Work out the finished part from the listing and answer in its coordinate system (mm). Face numbers are marked on the shaded views. Round coordinates to 2 decimals unless told otherwise and drop trailing zeros. Write each loop counter-clockwise with the first axis right and the second up, starting at its lowest first coordinate (ties: lowest second). Pieces come first, ordered by that corner, then holes. Notation, with made-up numbers: (33.5, -3) -> (65.5, -3) arc R19 ccw to (65.5, 21) -> close; hole circle Ø1 at (18, -13). An arc over 180 degrees is marked (long way). One line per item, written item: value.
```python
from build123d import *

# Parameters (mm, degrees)
SKETCH1_R           = 0.5
SKETCH1_R_2         = 0.25
SKETCH1_R_3         = 0.203
SKETCH1_R_4         = 1.25
BOSS_EXTRUDE1_DEPTH = 1.57
SKETCH2_R           = 1.758
SKETCH2_R_2         = 1.25
BOSS_EXTRUDE2_DEPTH = 0.0254
SKETCH3_R           = 0.881
SKETCH3_R_2         = 0.5
BOSS_EXTRUDE3_DEPTH = 0.0254


with BuildPart() as part:
    # Sketch1 → Boss-Extrude1 (new body)
    with BuildSketch(Plane(origin=(0, 0, 0), x_dir=(-1, 0, 0), z_dir=(0, 0, -1))):
        with BuildLine():
            Line((-22.86, 0), (-2.54, 0))
            ThreePointArc((-2.54, 0), (-0.743948776, 0.743948776), (0, 2.54))
            Line((0, 2.54), (0, 20.32))
            ThreePointArc((0, 20.32), (-0.743948776, 22.116051224), (-2.54, 22.86))
            Line((-2.54, 22.86), (-22.86, 22.86))
            ThreePointArc((-22.86, 22.86), (-24.656051224, 22.116051224), (-25.4, 20.32))
            Line((-25.4, 20.32), (-25.4, 2.54))
            ThreePointArc((-25.4, 2.54), (-24.656051224, 0.743948776), (-22.86, 0))
        make_face()
        with Locations(Location((-22.86, 2.54, 0), (0, 0, 180))):
            Circle(SKETCH1_R, mode=Mode.SUBTRACT)
        with Locations(Location((-17.78, 2.54, 0), (0, 0, 180))):
            Circle(SKETCH1_R, mode=Mode.SUBTRACT)
        with Locations(Location((-12.7, 2.54, 0), (0, 0, 180))):
            Circle(SKETCH1_R, mode=Mode.SUBTRACT)
        with Locations(Location((-7.62, 2.54, 0), (0, 0, 180))):
            Circle(SKETCH1_R, mode=Mode.SUBTRACT)
        with Locations(Location((-2.54, 2.54, 0), (0, 0, 180))):
            Circle(SKETCH1_R, mode=Mode.SUBTRACT)
        with Locations(Location((-7.874, 20.32, 0), (0, 0, 180))):
            Circle(SKETCH1_R_2, mode=Mode.SUBTRACT)
        with Locations(Location((-10.922, 15.24, 0), (0, 0, 180))):
            Circle(SKETCH1_R_2, mode=Mode.SUBTRACT)
        with Locations(Location((-11.684, 12.192, 0), (0, 0, 180))):
            Circle(SKETCH1_R_2, mode=Mode.SUBTRACT)
        with Locations(Location((-17.285, 13.462, 0), (0, 0, 180))):
            Circle(SKETCH1_R_3, mode=Mode.SUBTRACT)
        with Locations(Location((-20.828, 18.288, 0), (0, 0, 180))):
            Circle(SKETCH1_R_2, mode=Mode.SUBTRACT)
        with Locations(Location((-5.842, 15.494, 0), (0, 0, 180))):
            Circle(SKETCH1_R_2, mode=Mode.SUBTRACT)
        with Locations(Location((-16.256, 16.002, 0), (0, 0, 180))):
            Circle(SKETCH1_R_2, mode=Mode.SUBTRACT)
        with Locations(Location((-19.558, 13.462, 0), (0, 0, 180))):
            Circle(SKETCH1_R_3, mode=Mode.SUBTRACT)
        with Locations(Location((-11.938, 13.716, 0), (0, 0, 180))):
            Circle(SKETCH1_R_2, mode=Mode.SUBTRACT)
        with Locations(Location((-2.54, 20.32, 0), (0, 0, 180))):
            Circle(SKETCH1_R_4, mode=Mode.SUBTRACT)
        with Locations(Location((-22.86, 20.32, 0), (0, 0, 180))):
            Circle(SKETCH1_R_4, mode=Mode.SUBTRACT)
        with Locations(Location((-5.08, 2.54, 0), (0, 0, 180))):
            Circle(SKETCH1_R, mode=Mode.SUBTRACT)
        with Locations(Location((-10.16, 2.54, 0), (0, 0, 180))):
            Circle(SKETCH1_R, mode=Mode.SUBTRACT)
        with Locations(Location((-15.24, 2.54, 0), (0, 0, 180))):
            Circle(SKETCH1_R, mode=Mode.SUBTRACT)
        with Locations(Location((-20.32, 2.54, 0), (0, 0, 180))):
            Circle(SKETCH1_R, mode=Mode.SUBTRACT)
    extrude(amount=-BOSS_EXTRUDE1_DEPTH)

    # Sketch2 → Boss-Extrude2 (add)
    # profile 1 of 2: a face of its own
    with BuildSketch(Plane.XY.offset(1.57)):
        with Locations(Location((2.54, 20.32, 0), (0, 0, 180))):
            Circle(SKETCH2_R)
        with Locations((2.54, 20.32)):
            Circle(SKETCH2_R_2, mode=Mode.SUBTRACT)
    # profile 2 of 2: a face of its own
    with BuildSketch(Plane.XY.offset(1.57)):
        with Locations(Location((22.86, 20.32, 0), (0, 0, 180))):
            Circle(SKETCH2_R)
        with Locations((22.86, 20.32)):
            Circle(SKETCH2_R_2, mode=Mode.SUBTRACT)
    boss_extrude2 = extrude(amount=BOSS_EXTRUDE2_DEPTH)

    # Mirror1: Boss-Extrude2 across plane
    add(boss_extrude2.mirror(Plane.XY.offset(0.785)))

    # Sketch3 → Boss-Extrude3 (add)
    # profile 1 of 9: a face of its own
    with BuildSketch(Plane.XY.offset(1.57)):
        with Locations(Location((2.54, 2.54, 0), (0, 0, 180))):
            Circle(SKETCH3_R)
        with Locations((2.54, 2.54)):
            Circle(SKETCH3_R_2, mode=Mode.SUBTRACT)
    # profile 2 of 9: a face of its own
    with BuildSketch(Plane.XY.offset(1.57)):
        with Locations(Location((5.08, 2.54, 0), (0, 0, 180))):
            Circle(SKETCH3_R)
        with Locations((5.08, 2.54)):
            Circle(SKETCH3_R_2, mode=Mode.SUBTRACT)
    # profile 3 of 9: a face of its own
    with BuildSketch(Plane.XY.offset(1.57)):
        with Locations(Location((7.62, 2.54, 0), (0, 0, 180))):
            Circle(SKETCH3_R)
        with Locations((7.62, 2.54)):
            Circle(SKETCH3_R_2, mode=Mode.SUBTRACT)
    # profile 4 of 9: a face of its own
    with BuildSketch(Plane.XY.offset(1.57)):
        with Locations(Location((10.16, 2.54, 0), (0, 0, 180))):
            Circle(SKETCH3_R)
        with Locations((10.16, 2.54)):
            Circle(SKETCH3_R_2, mode=Mode.SUBTRACT)
    # profile 5 of 9: a face of its own
    with BuildSketch(Plane.XY.offset(1.57)):
        with Locations(Location((12.7, 2.54, 0), (0, 0, 180))):
            Circle(SKETCH3_R)
        with Locations((12.7, 2.54)):
            Circle(SKETCH3_R_2, mode=Mode.SUBTRACT)
    # profile 6 of 9: a face of its own
    with BuildSketch(Plane.XY.offset(1.57)):
        with Locations(Location((15.24, 2.54, 0), (0, 0, 180))):
            Circle(SKETCH3_R)
        with Locations((15.24, 2.54)):
            Circle(SKETCH3_R_2, mode=Mode.SUBTRACT)
    # profile 7 of 9: a face of its own
    with BuildSketch(Plane.XY.offset(1.57)):
        with Locations(Location((17.78, 2.54, 0), (0, 0, 180))):
            Circle(SKETCH3_R)
        with Locations((17.78, 2.54)):
            Circle(SKETCH3_R_2, mode=Mode.SUBTRACT)
    # profile 8 of 9: a face of its own
    with BuildSketch(Plane.XY.offset(1.57)):
        with Locations(Location((20.32, 2.54, 0), (0, 0, 180))):
            Circle(SKETCH3_R)
        with Locations((20.32, 2.54)):
            Circle(SKETCH3_R_2, mode=Mode.SUBTRACT)
    # profile 9 of 9: a face of its own
    with BuildSketch(Plane.XY.offset(1.57)):
        with Locations(Location((22.86, 2.54, 0), (0, 0, 180))):
            Circle(SKETCH3_R)
        with Locations((22.86, 2.54)):
            Circle(SKETCH3_R_2, mode=Mode.SUBTRACT)
    boss_extrude3 = extrude(amount=BOSS_EXTRUDE3_DEPTH)

    # Mirror2: Boss-Extrude3 across plane
    add(boss_extrude3.mirror(Plane.XY.offset(0.785)))


solid = part.part
```
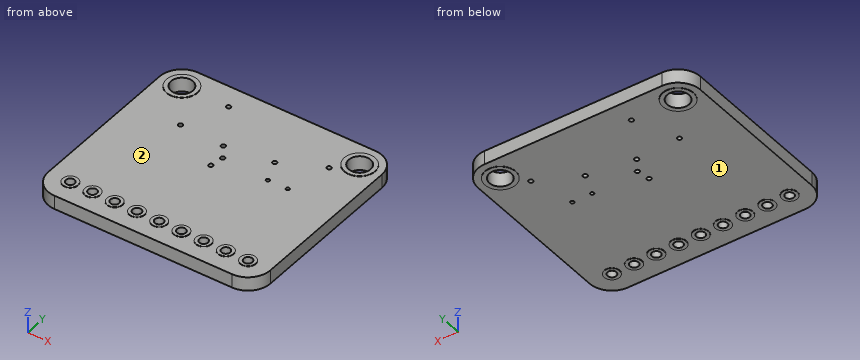
(1) Flat-ended cylindrical pins translate along their axes: pin 1 Ø7 at (x, y) = (9, 6.5) entering from +Z; pin 2 Ø2 at (x, y) = (12, 12.5) entering from -Z. Find the tip coordinate at first contact, or state that the pin passes through.
Reported:
pin 1: stops at z = 1.6
pin 2: stops at z = 0
(2) Find section B-B on y = 19.5. Give the number of separate pieces and of enclosed holes in the cut face, plus the area to 3 significant figures.
Reported:
separate pieces: 3
enclosed holes: 0
area: 34.1 mm2
(3) Find section D-D on y = 4.25. Give the vertices of the cut face in (x, z).
Reported:
outline: (0, 0) -> (25.4, 0) -> (25.4, 1.57) -> (0, 1.57) -> close
(4) Consider probe 1 along X at (y, z) = (20.32, 1.05); probe 2 along Y at (x, z) = (2.54, 0.6); probe 3 along Y at (x, z) = (20.32, 0.95). Determine where each line is inside the solid, lowest interval first.
Reported:
probe 1: x = 0 to 1.29, 3.79 to 7.62, 8.12 to 21.61, 24.11 to 25.4
probe 2: y = 0 to 2.04, 3.04 to 19.07, 21.57 to 22.86
probe 3: y = 0 to 2.04, 3.04 to 22.86
(5) For a pull along X with two mould halves and no side action, classify the marked faces 1 and 2 as pulls with the +X half, pulls with the -X half, needs draft (parallel to the pull), parting line crosses it, or undercut.
Reported:
face 1: undercut
face 2: undercut
